Input: part model. Units: mm. Frame: model coordinates. A direction names the side the tool comes from. Coordinates: 2 decimals unless noted, no trailing zeros. Loops run counter-clockwise (first coordinate to the right, second up) from the corner with the lowest first, then second, coordinate; pieces in that order, holes last. Notation, with made-up numbers: (-4, 38) - (45, 38) arc R19 cw to (45, 68) - close; hole circle Ø4 at (-36.5, 89.5). An arc over 180 degrees is marked (long way). Use one line per item in the form item = value.
from build123d import *

# Parameters (mm, degrees)
SKETCH1_R           = 6.375
SKETCH1_R_2         = 4.875
BOSS_EXTRUDE1_DEPTH = 50
SKETCH2_W           = 2.1
SKETCH2_H           = 10
CUT_EXTRUDE1_DEPTH  = 13.75
CUT_EXTRUDE2_DEPTH  = 13.75
FILLET1_R           = 1
CHAMFER1_SIZE       = 0.5
SKETCH4_R           = 2.5
CUT_EXTRUDE3_DEPTH  = 13.7500001


with BuildPart() as part:
    # Sketch1 → Boss-Extrude1 (new body)
    with BuildSketch(Plane(origin=(0, 0, 0), x_dir=(1, 0, 0), z_dir=(0, 1, 0))):
        Circle(SKETCH1_R)
        Circle(SKETCH1_R_2, mode=Mode.SUBTRACT)
    extrude(amount=BOSS_EXTRUDE1_DEPTH)

    # Sketch2 → Cut-Extrude1 (cut, through all)
    with BuildSketch(Plane(origin=(0, 0, -6.375), x_dir=(-1, 0, 0), z_dir=(0, 0, -1))):
        with Locations((0, 5)):
            Rectangle(SKETCH2_W, SKETCH2_H)
    extrude(amount=-CUT_EXTRUDE1_DEPTH, mode=Mode.SUBTRACT)

    # Sketch3 → Cut-Extrude2 (cut, through all)
    with BuildSketch(Plane(origin=(0, 0, -6.375), x_dir=(-1, 0, 0), z_dir=(0, 0, -1))):
        Polygon((2.05, 0), (-2.05, 0), (0, 2.05), align=None)
    extrude(amount=-CUT_EXTRUDE2_DEPTH, mode=Mode.SUBTRACT)

    # Fillet1
    fillet1_edges = [part.edges().sort_by_distance(p)[0] for p in [
        (-1.05, 10, -5.524257599),
        (-1.05, 10, 5.524257599),
        (1.05, 10, -5.524257599),
        (1.05, 10, 5.524257599),
    ]]
    fillet(fillet1_edges, radius=FILLET1_R)

    # Chamfer1
    chamfer1_edges = [part.edges().sort_by_distance(p)[0] for p in [
        (5.182150857, 0, -3.712941893),
        (-6.375, 0, 0),
        (-6.375, 50, 0),
    ]]
    chamfer(chamfer1_edges, length=CHAMFER1_SIZE)

    # Sketch4 → Cut-Extrude3 (cut, through all)
    with BuildSketch(Plane(origin=(0, 0, -6.375), x_dir=(-1, 0, 0), z_dir=(0, 0, -1))):
        with Locations((0, 40)):
            Circle(SKETCH4_R)
    extrude(amount=-CUT_EXTRUDE3_DEPTH, mode=Mode.SUBTRACT)


solid = part.part
Q1. Cut plane C-C, the plane x = -0.5. Give the number of separate pieces and of enclosed holes in the cut face, then the cut area to 3 significant figures.
Check values:
separate_pieces = 4
enclosed_holes = 0
area = 106 mm²
Q2. Ray query, line 1 along X through (y, z) = (31, 0) (3 decimals); line 2 along Y through (x, z) = (0, -5); line 3 along X through (y, z) = (30, 2.5). Return the intervals inside material, ascending. Write a range as [from, to].
Check values:
line_1 = [-6.375, -4.875], [4.875, 6.375]
line_2 = [10, 37.5], [42.5, 50]
line_3 = [-5.86, -4.19], [4.19, 5.86]
Q3. Cut plane B-B, the plane y = 40. Return loops of the section in (x, z) (3 decimals).
Check values:
outline = (-2.5, -5.864) - (-2.5, -4.185) arc R4.875 cw to (-2.5, 4.185) - (-2.5, 5.864) arc R6.375 ccw to start; (2.5, -5.864) arc R6.375 ccw to (2.5, 5.864) - (2.5, 4.185) arc R4.875 cw to (2.5, -4.185) - close
Q4. Set-up query: faces 4 (the cylindrical face through (0.749, 9.715, 5.579)), 5 (the cylindrical face through (2, 38.5, 5.3)). Return all of +Z, -Z, +X, -X, +Y, -Y with unobstructed straight access to the full face (end or side cutting, diameter ignored); none if empty.
Check values:
face_4 = +Z, -Z, -Y
face_5 = +Z, -Z
Q5. Cut plane D-D, the plane y = 15. Return loops of the section in (x, z) (3 decimals).
Check values:
outline = circle Ø12.75 at (0, 0); hole circle Ø9.75 at (0, 0)
Q6. First-contact query: P1, Ø1.5, axis at x = 1.5, y = 29, coming from the -Z side; P2, Ø0.5, axis at y = 5, z = 5.5, coming from the -X side; P3, Ø4, axis at y = 44.5, z = -2.5, coming from the -X side. Flat tips, straight axial feed; report the tip coordinate or a pass-through.
Check values:
P1 = -6.33
P2 = -3.62
P3 = -6.36
Q7. Cut plane A-A, the plane z = 0. Return loops of the section in (x, y) (3 decimals), then the cut area to 4 significant figures.
Check values:
outline = (-6.375, 0.5) - (-5.875, 0) - (-4.875, 0) - (-4.875, 50) - (-5.875, 50) - (-6.375, 49.5) - close; (4.875, 0) - (5.875, 0) - (6.375, 0.5) - (6.375, 49.5) - (5.875, 50) - (4.875, 50) - close
area = 149.5 mm²
Q8. Pull-direction query (X, two-part tool) for faces 1 (the flat face through (-5.1, 0, 0.4)), 2 (the flat face through (-1.54, 0.51, -5.37)), 3 (the conical face through (-6.009, 0.135, -0.112)); classes: pulls with the +X half, pulls with the -X half, needs draft (parallel to the pull), parting line crosses it, or undercut.
Check values:
face_1 = needs draft
face_2 = undercut
face_3 = pulls with the -X half
